```python
from build123d import *

# Parameters (mm, degrees)
SKETCH1_R                                       = 29.692527183
SKETCH1_R_2                                     = 22.692527183
SKETCH1_R_3                                     = 19.692527183
SKETCH1_R_4                                     = 16.692527183
BOSS_EXTRUDE1_DEPTH                             = 5
CSK_FOR_M3_FLAT_HEAD_MACHINE_SCREW2_D           = 3.4
CSK_FOR_M3_FLAT_HEAD_MACHINE_SCREW2_DEPTH       = 12
CSK_FOR_M3_FLAT_HEAD_MACHINE_SCREW2_CSINK_D     = 7.3
CSK_FOR_M3_FLAT_HEAD_MACHINE_SCREW2_CSINK_ANGLE = 90
CSK_FOR_M3_FLAT_HEAD_MACHINE_SCREW2_TIP         = 1.021463052
SKETCH9_W                                       = 27.5
SKETCH9_H                                       = 28
BOSS_EXTRUDE2_DEPTH                             = 7.5
SKETCH10_W                                      = 23.5
SKETCH10_H                                      = 25.45
CUT_EXTRUDE1_DEPTH                              = 6.1
SKETCH12_W                                      = 6
SKETCH12_H                                      = 11
CUT_EXTRUDE2_DEPTH                              = 3
CUT_EXTRUDE3_REACH                              = 55.407
SKETCH11_W                                      = 9.585282086
SKETCH11_H                                      = 9.717675131


with BuildPart() as part:
    # Sketch1 → Boss-Extrude1 (new body)
    # profile 1 of 4: a face of its own
    with BuildSketch(Plane(origin=(0, 0, 0), x_dir=(-1, 0, 0), z_dir=(0, 0, 1))):
        with Locations(Location((0, 0, 0), (0, 0, 180))):
            Circle(SKETCH1_R)
        Circle(SKETCH1_R_2, mode=Mode.SUBTRACT)
    # profile 2 of 4: a face of its own
    with BuildSketch(Plane(origin=(0, 0, 0), x_dir=(-1, 0, 0), z_dir=(0, 0, 1))):
        Circle(SKETCH1_R_2)
        Circle(SKETCH1_R_3, mode=Mode.SUBTRACT)
    # profile 3 of 4: a face of its own
    with BuildSketch(Plane(origin=(0, 0, 0), x_dir=(-1, 0, 0), z_dir=(0, 0, 1))):
        Circle(SKETCH1_R_3)
        Circle(SKETCH1_R_4, mode=Mode.SUBTRACT)
    # profile 4 of 4: a face of its own
    with BuildSketch(Plane(origin=(0, 0, 0), x_dir=(-1, 0, 0), z_dir=(0, 0, 1))):
        with BuildLine():
            Line((14.058465911, 9), (-14.058465911, 9))
            ThreePointArc((-14.058465911, 9), (-16.692527183, 0), (-14.058465911, -9))
            Line((-14.058465911, -9), (14.058465911, -9))
            ThreePointArc((14.058465911, -9), (16.020483578, -4.688770595), (16.692527183, 0))
            ThreePointArc((16.692527183, 0), (16.020483578, 4.688770595), (14.058465911, 9))
        make_face()
    extrude(amount=BOSS_EXTRUDE1_DEPTH)

    # CSK for M3 Flat Head Machine Screw2
    with Locations(Plane.XY.offset(5)):
        with Locations((0, 19.692527183), (0, -19.692527183), (19.692527183, 0), (-19.692527183, 0)):
            CounterSinkHole(CSK_FOR_M3_FLAT_HEAD_MACHINE_SCREW2_D / 2, CSK_FOR_M3_FLAT_HEAD_MACHINE_SCREW2_CSINK_D / 2, depth=CSK_FOR_M3_FLAT_HEAD_MACHINE_SCREW2_DEPTH, counter_sink_angle=CSK_FOR_M3_FLAT_HEAD_MACHINE_SCREW2_CSINK_ANGLE)
            with Locations((0, 0, -(CSK_FOR_M3_FLAT_HEAD_MACHINE_SCREW2_DEPTH + CSK_FOR_M3_FLAT_HEAD_MACHINE_SCREW2_TIP / 2))):  # 118° drill point
                Cone(0, CSK_FOR_M3_FLAT_HEAD_MACHINE_SCREW2_D / 2, CSK_FOR_M3_FLAT_HEAD_MACHINE_SCREW2_TIP, mode=Mode.SUBTRACT)

    # Sketch9 → Boss-Extrude2 (add, symmetric)
    with BuildSketch(Plane(origin=(0, 0, 0), x_dir=(1, 0, 0), z_dir=(0, 1, 0))):
        with Locations((0, 14)):
            Rectangle(SKETCH9_W, SKETCH9_H)
    extrude(amount=BOSS_EXTRUDE2_DEPTH, both=True)

    # Sketch10 → Cut-Extrude1 (cut, symmetric)
    with BuildSketch(Plane(origin=(0, 0, 0), x_dir=(1, 0, 0), z_dir=(0, 1, 0))):
        with Locations((0, 12.775)):
            Rectangle(SKETCH10_W, SKETCH10_H)
    extrude(amount=CUT_EXTRUDE1_DEPTH, both=True, mode=Mode.SUBTRACT)

    # Sketch12 → Cut-Extrude2 (cut)
    with BuildSketch(Plane.XY.offset(-28)):
        with Locations((8.75, 0)):
            Rectangle(SKETCH12_W, SKETCH12_H)
    extrude(amount=CUT_EXTRUDE2_DEPTH, mode=Mode.SUBTRACT)

    # Cut-Extrude3: up to this face of the body (flat: up to its plane)
    cut_extrude3_end = Plane(part.part.faces().sort_by_distance((0, 0, -0.05))[0])
    # Sketch11 → Cut-Extrude3 (cut, up to the picked face)
    with BuildSketch(Plane.XY.offset(5), mode=Mode.PRIVATE) as cut_extrude3_sk1:
        with Locations((8.957358957, -0.433824782)):
            Rectangle(SKETCH11_W, SKETCH11_H)
    cut_extrude3_tool1 = split(extrude(cut_extrude3_sk1.sketch, amount=-CUT_EXTRUDE3_REACH, mode=Mode.PRIVATE), bisect_by=cut_extrude3_end, keep=Keep.BOTH, mode=Mode.PRIVATE)
    add(cut_extrude3_tool1.solids().sort_by(Axis((8.957359, -0.433825, 5), (0, 0, -1)))[0], mode=Mode.SUBTRACT)


solid = part.part
```
Part model, mm, in its own coordinate system. A direction names the side the tool comes from. Round coordinates to 2 decimals unless told otherwise and drop trailing zeros. Loops run counter-clockwise (first coordinate to the right, second up) from the corner with the lowest first, then second, coordinate; pieces in that order, holes last.
1. Slice it at C-C (z = -19.5). Give the cut face in (x, y), and give its area (3 significant figures).
Solutions:
outline: (-13.75, -7.5) - (13.75, -7.5) - (13.75, 7.5) - (-13.75, 7.5) - close; hole (-11.75, -6.1) - (11.75, -6.1) - (11.75, 6.1) - (-11.75, 6.1) - close
area: 126 mm2
2. Drill centre lines: line 1 along Y through (x, z) = (0, 1.6); line 2 along Y through (x, z) = (11, -11.5); line 3 along Z through (x, y) = (-11, 8.5). Where is each one in solid material? Low to high.
Solutions:
line 1: y = -29.69 to -21.39, -17.99 to -16.69, -9 to 9, 16.69 to 17.99, 21.39 to 29.69
line 2: y = -7.5 to -6.1, 6.1 to 7.5
line 3: z = 0 to 5
3. Two-plate mould, pull along Y, no slides. Class faces 4 (the face through (0, 7.5, -14)), 5 (the face through (0, -6.1, -13)), 6 (the face through (-13, 13, 0)): pulls with the +Y half, pulls with the -Y half, needs draft (parallel to the pull), parting line crosses it, or undercut.
Solutions:
face 4: pulls with the +Y half
face 5: undercut
face 6: needs draft
4. Slice it at A-A (x = 0). Count the separate pieces of the cut face and the enclosed holes in it, and give its area (3 significant figures).
Solutions:
separate pieces: 5
enclosed holes: 1
area: 288 mm2
5. Flat gauge pins, fed straight in: pin 1 (19 mm diameter, centred on x = 1, z = -11, fed in from -Y); pin 2 (2 mm diameter, centred on x = 0, y = -19.69, fed in from -Z); pin 3 (7 mm diameter, centred on x = -3, z = -13.5, fed in from +Y); pin 4 (2 mm diameter, centred on x = 21, y = 8, fed in from -Z). Where does each tip first touch, or does it go through?
Solutions:
pin 1: stops at y = -7.5
pin 2: passes through
pin 3: stops at y = 7.5
pin 4: stops at z = 0
6. 3-axis set-ups, long thin cutter, end or side, ignore diameter. For faces 1 (the face through (0, -9, 2)), 2 (the face through (-11.75, 0, -13)), 3 (the face through (4.165, -1, 3)): which of +Z, -Z, +X, -X, +Y, -Y reach the whole face in a straight line?
Solutions:
face 1: +Z, -Z
face 2: none
face 3: +Z
7. Slice it at D-D (y = 14.5). Give the cut face in (x, z), and give its area (3 significant figures).
Solutions:
outline: (-25.91, 0) - (-8.27, 0) - (-8.27, 5) - (-25.91, 5) - close; (8.27, 0) - (25.91, 0) - (25.91, 5) - (8.27, 5) - close
area: 176 mm2
